For this review, take the finished solid that the model builds, in its own axes (mm). A direction names the side the tool comes from. Give positions to 0.01 mm unless a question says otherwise; leave off trailing zeros. Write each loop counter-clockwise with the first axis right and the second up, starting at its lowest first coordinate (ties: lowest second). Pieces come first, ordered by that corner, then holes.
Q1. We need section A-A (z = 2294.5). Write out the cut boundary in (x, y).
Q2. We need section B-B (z = 2834). Write out the cut boundary in (x, y).
Q3. We need section C-C (z = 2610). Write out the cut boundary in (x, y), then the cut area to 3 significant figures.
Q4. For line 1 (Z direction, x = -9.5, y = 16); line 2 (Z direction, x = 23, y = 28.5); line 3 (X direction, y = 16, z = 2676), list the stretches that pass through material, from the lowest coordinate up.
Q5. Machinability: for faces 4 (the flat face through (32.366, 6, 2497)), 5 (the flat face through (26, 23, 2750.359)), 6 (the flat face through (18, 9.837, 2829)), 7 (the flat face through (1, 7, 2735.359)), which of the approach directions +Z, -Z, +X, -X, +Y, -Y give a long, thin tool a straight path to every point of the face, cutting with its end or side? Answer none if there is none.
Q6. Insertion check: P1, Ø5, axis at x = 6.37, y = 6.34, coming from the -Z side; P2, Ø1, axis at x = 41.5, y = 12, coming from the +Z side; P3, Ø5, axis at x = 43.87, y = 6.34, coming from the -Z side. Each pin has a flat end and moves straight along its axis. Give the tip position at first contact, or say it passes through.
Q7. Mouldability with a two-part tool opening along Y and no side actions: class faces 1 (the flat face through (17, 17, 2755.359)), 2 (the flat face through (-19.634, 11, 2580)), 3 (the flat face through (11, -6.163, 2580)) as released by +Y, released by -Y, zero draft, split by the parting line, or undercut.
```python
from build123d import *

# Parameters (mm, degrees)
SKETCH1_W                = 520
SKETCH1_H                = 250
BOSS_EXTRUDE1_DEPTH      = 5000
SKETCH2_W                = 450
SKETCH2_H                = 250
CUT_EXTRUDE1_DEPTH       = 600
SKETCH3_W                = 750
SKETCH3_H                = 470
BOSS_EXTRUDE2_DEPTH      = 50
SKETCH4_R                = 32.5
CUT_EXTRUDE2_DEPTH       = 50
CUT_EXTRUDE3_DEPTH       = 4937.509394299
CUT_EXTRUDE3_DEPTH_BACK  = 170
SKETCH5_R                = 30
SCALE2_SCALE             = 0.1
FILLET1_R                = 10
BOSS_EXTRUDE9_DEPTH      = 150
BOSS_EXTRUDE9_DEPTH_BACK = 1
CUT_EXTRUDE4_DEPTH       = 2907.266833376
CUT_EXTRUDE4_DEPTH_BACK  = 2907.266833376
SKETCH7_R                = 5
SKETCH8_R                = 3.25
CUT_EXTRUDE5_DEPTH       = 20


with BuildPart() as part:
    # Sketch1 → Boss-Extrude1 (new body)
    with BuildSketch(Plane.XY):
        Rectangle(SKETCH1_W, SKETCH1_H)
    extrude(amount=BOSS_EXTRUDE1_DEPTH)

    # Sketch2 → Cut-Extrude1 (cut)
    with BuildSketch(Plane.XY.offset(4850)):
        Rectangle(SKETCH2_W, SKETCH2_H)
    cut_extrude1 = extrude(amount=-CUT_EXTRUDE1_DEPTH, mode=Mode.SUBTRACT)

    # Mirror1: Cut-Extrude1 across plane
    add(cut_extrude1.mirror(Plane.XY.offset(2500)), mode=Mode.SUBTRACT)

    # Sketch3 → Boss-Extrude2 (add)
    with BuildSketch(Plane.XY.offset(5000)):
        with Locations((115, 110)):
            Rectangle(SKETCH3_W, SKETCH3_H)
    boss_extrude2 = extrude(amount=BOSS_EXTRUDE2_DEPTH)

    # Sketch4 → Cut-Extrude2 (cut)
    with BuildSketch(Plane.XY.offset(5050)):
        with Locations((375, 0)):
            Circle(SKETCH4_R)
        with Locations((360, 255)):
            Circle(SKETCH4_R)
    cut_extrude2 = extrude(amount=-CUT_EXTRUDE2_DEPTH, mode=Mode.SUBTRACT)

    # Mirror2: Boss-Extrude2, Cut-Extrude2 across plane
    add(boss_extrude2.mirror(Plane.XY.offset(2500)))
    add(cut_extrude2.mirror(Plane.XY.offset(2500)), mode=Mode.SUBTRACT)

    # Sketch5 → Cut-Extrude3 (cut, two sides: drawn at the far end of the back side and taken through both)
    with BuildSketch(Plane(origin=(0, 0, 4850), x_dir=(-1, 0, 0), z_dir=(0, 0, -1)).offset(-CUT_EXTRUDE3_DEPTH_BACK)):
        with Locations(Location((0, 0, 0), (0, 0, 180))):
            Circle(SKETCH5_R)
    extrude(amount=CUT_EXTRUDE3_DEPTH + CUT_EXTRUDE3_DEPTH_BACK, mode=Mode.SUBTRACT)


with BuildPart() as part_1:
    # Scale2: scaled about (7.073044916, 7.041537563, 2500.399199176)
    add(part.part.scale(SCALE2_SCALE).moved(Location((6.365740424, 6.337383807, 2250.359279258))))

    # Fillet1
    # the kernel refuses this fillet: 10 mm, written as the material it takes off along each edge
    with BuildSketch(Plane(origin=(-19.634259576, 40.837383807, 2725.359279258), x_dir=(0, -1, 0), z_dir=(0, 0, 1)), Plane(origin=(55.365740424, 40.837383807, 2725.359279258), x_dir=(-1, 0, 0), z_dir=(0, 0, 1)), Plane(origin=(55.365740424, -6.162616193, 2275.359279258), x_dir=(-1, 0, 0), z_dir=(0, 0, -1))) as fillet1_piece_1:
        with BuildLine():
            CenterArc((FILLET1_R, FILLET1_R), FILLET1_R, 180, 90)
            Line((0, FILLET1_R), (0, 0))
            Line((0, 0), (FILLET1_R, 0))
        make_face()
    extrude(amount=55, mode=Mode.SUBTRACT)
    with BuildSketch(Plane(origin=(55.365740424, -6.162616193, 2725.359279258), x_dir=(-1, 0, 0), z_dir=(0, 0, 1)), Plane(origin=(-19.634259576, 40.837383807, 2275.359279258), x_dir=(0, -1, 0), z_dir=(0, 0, -1)), Plane(origin=(55.365740424, 40.837383807, 2275.359279258), x_dir=(-1, 0, 0), z_dir=(0, 0, -1))) as fillet1_piece_2:
        with BuildLine():
            CenterArc((FILLET1_R, -FILLET1_R), FILLET1_R, 90, 90)
            Line((0, -FILLET1_R), (0, 0))
            Line((0, 0), (FILLET1_R, 0))
        make_face()
    extrude(amount=55, mode=Mode.SUBTRACT)
    with BuildSketch(Plane(origin=(-19.634259576, -6.162616193, 2220.359279258), x_dir=(0, 1, 0), z_dir=(0, 0, 1))) as fillet1_piece_3:
        with BuildLine():
            CenterArc((FILLET1_R, -FILLET1_R), FILLET1_R, 90, 90)
            Line((0, -FILLET1_R), (0, 0))
            Line((0, 0), (FILLET1_R, 0))
        make_face()
    extrude(amount=560, mode=Mode.SUBTRACT)

    # Sketch6 → Boss-Extrude9 (add, two sides: drawn at the far end of the back side and taken through both)
    with BuildSketch(Plane.XY.offset(2755.359279258).offset(-BOSS_EXTRUDE9_DEPTH_BACK)):
        with BuildLine():
            Line((-9.634259575, -6.162616194), (45.365740425, -6.162616194))
            ThreePointArc((45.365740425, -6.162616194), (52.436808237, -3.233684006), (55.365740425, 3.837383806))
            Line((55.365740425, 3.837383806), (55.365740425, 9.837383806))
            Line((55.365740425, 9.837383806), (-19.634259575, 9.837383806))
            Line((-19.634259575, 9.837383806), (-19.634259575, 3.837383806))
            ThreePointArc((-19.634259575, 3.837383806), (-16.705327387, -3.233684006), (-9.634259575, -6.162616194))
        make_face()
        with BuildLine():
            Line((-9.634259575, 40.837383806), (45.365740425, 40.837383806))
            ThreePointArc((45.365740425, 40.837383806), (52.436808237, 37.908451618), (55.365740425, 30.837383806))
            Line((55.365740425, 30.837383806), (55.365740425, 24.837383806))
            Line((55.365740425, 24.837383806), (-19.634259575, 24.837383806))
            Line((-19.634259575, 24.837383806), (-19.634259575, 30.837383806))
            ThreePointArc((-19.634259575, 30.837383806), (-16.705327387, 37.908451618), (-9.634259575, 40.837383806))
        make_face()
    extrude(amount=BOSS_EXTRUDE9_DEPTH + BOSS_EXTRUDE9_DEPTH_BACK)

    # Sketch7 → Cut-Extrude4 (cut, two sides: drawn at the far end of the back side and taken through both)
    with BuildSketch(Plane(origin=(0, 40.837383806, 0), x_dir=(1, 0, 0), z_dir=(0, 1, 0)).offset(-CUT_EXTRUDE4_DEPTH_BACK)):
        with Locations(Location((17.865740425, -2880.359279258, 0), (0, 0, 270))):
            Circle(SKETCH7_R)
    extrude(amount=CUT_EXTRUDE4_DEPTH + CUT_EXTRUDE4_DEPTH_BACK, mode=Mode.SUBTRACT)

    # Sketch8 → Cut-Extrude5 (cut)
    with BuildSketch(Plane(origin=(0, 0, 2754.359279258), x_dir=(-1, 0, 0), z_dir=(0, 0, -1))):
        with Locations(Location((-42.365740425, 31.837383806, 0), (0, 0, 180))):
            Circle(SKETCH8_R)
        with Locations(Location((-43.865740425, 6.337383806, 0), (0, 0, 180))):
            Circle(SKETCH8_R)
    extrude(amount=-CUT_EXTRUDE5_DEPTH, mode=Mode.SUBTRACT)


solid = part_1.part
```
Computed:
1. outline: (-19.63, 3.84) arc R10 ccw to (-16.13, -3.76) - (-16.13, 18.84) - (-19.63, 18.84) - close; (28.87, -6.16) - (32.37, -6.16) - (32.37, 18.84) - (28.87, 18.84) - close
2. outline: (-19.63, 3.84) arc R10 ccw to (-9.63, -6.16) - (45.37, -6.16) arc R10 ccw to (55.37, 3.84) - (55.37, 9.84) - (-19.63, 9.84) - close; (-19.63, 24.84) - (55.37, 24.84) - (55.37, 30.84) arc R10 ccw to (45.37, 40.84) - (-9.63, 40.84) arc R10 ccw to (-19.63, 30.84) - close
3. outline: (-19.63, 3.84) arc R10 ccw to (-9.63, -6.16) - (32.37, -6.16) - (32.37, 18.84) - (-19.63, 18.84) - close; hole circle Ø6 at (6.37, 6.34)
3. area: 1,250 mm2
4. line 1: z = 2245.36 to 2265.36, 2325.36 to 2675.36, 2735.36 to 2755.36
4. line 2: z = 2245.36 to 2250.36, 2750.36 to 2905.36
4. line 3: x = -19.63 to -16.13, 28.87 to 32.37
5. face 4: +X, +Y, -Y
5. face 5: +X, +Y
5. face 6: +Z, +X, -X
5. face 7: +Y, -Y
6. P1: stops at z = 2752.36
6. P2: stops at z = 2755.36
6. P3: stops at z = 2774.36
7. face 1: undercut
7. face 2: zero draft
7. face 3: released by -Y
